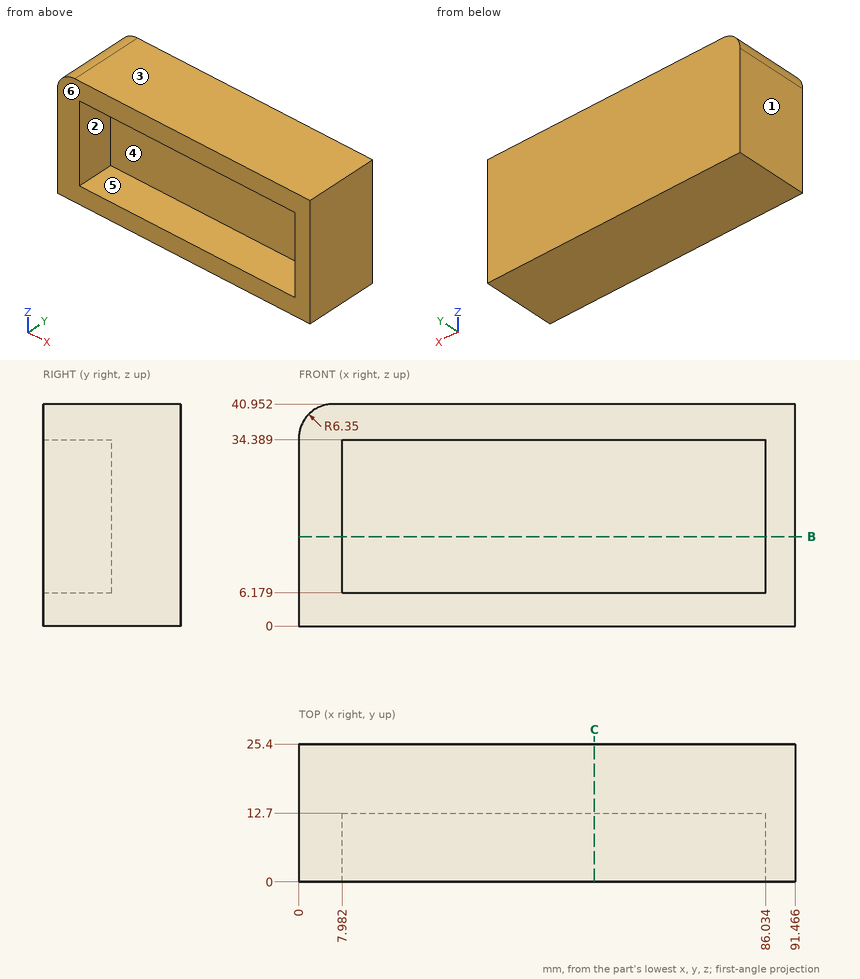
For this review, use the dimensioned drawing (mm, ordinates from the lowest corner) and the shaded views. A direction names the side the tool comes from. Give positions to 0.01 mm unless a question says otherwise; leave off trailing zeros. Order: outer loops, then holes, each group sorted by start corner. A loop starts at its lowest first (then second) coordinate and runs counter-clockwise, first axis right, second up.
1) Take a section at C-C (x = 54.5). Give the boundary of the cut face in (y, z).
2) Insertion check: pin 1 (4 mm diameter, centred on x = 16, z = 18.5, fed in from -Y). The pin has a flat end and moves straight along its axis. Give the tip position at first contact, or say it passes through.
3) Take a section at B-B (z = 16.5). Give the boundary of the cut face in (x, y) (1 decimal).
4) The part is to be moulded in two halves that separate along X. For the marked faces 1, 2, 3 and 4, say which applies: released by +X, released by -X, zero draft, split by the parting line, or undercut.
5) Wall thickness on line 1 (X direction, y = 8.25, z = 28.5) (1 decimal); line 2 (Z direction, x = 59, y = 11.5); line 3 (Y direction, x = 9.5, z = 16): over which ranges is each line inside the solid? List them lowest first.
6) For the marked faces 5 and 6, list the 3-axis set-ups (+Z, -Z, +X, -X, +Y, -Y) from which the entire face can be reached by the end or side of a thin tool; tool diameter is ignored.
Derived:
1. outline: (0, 0) - (25.4, 0) - (25.4, 40.95) - (0, 40.95) - (0, 34.39) - (12.7, 34.39) - (12.7, 6.18) - (0, 6.18) - close
2. pin 1: stops at y = 12.7
3. outline: (0, 0) - (8, 0) - (8, 12.7) - (86, 12.7) - (86, 0) - (91.5, 0) - (91.5, 25.4) - (0, 25.4) - close
4. face 1: released by -X
4. face 2: undercut
4. face 3: zero draft
4. face 4: undercut
5. line 1: x = 0 to 8, 86 to 91.5
5. line 2: z = 0 to 6.18, 34.39 to 40.95
5. line 3: y = 12.7 to 25.4
6. face 5: -Y
6. face 6: +Z, -Z, +X, -X, -Y
